from build123d import *

# Parameters (mm, degrees)
F0_R      = 66.728095
F1_DEPTH  = 12.7
F3_DEPTH  = 25.4
F5_DEPTH  = 25.4
F7_DEPTH  = 12.7
F9_DEPTH  = 25.4
F11_DEPTH = 6.35


with BuildPart() as f1:
    # F0 (on Top) → F1 (new body)
    with BuildSketch(Plane.XY):
        with Locations((-8.514826, -3.963798)):
            Circle(F0_R)
    extrude(amount=F1_DEPTH)

    # F2 (on face) → F3 (cut)
    with BuildSketch(Plane.XY.offset(12.7)):
        Polygon((-24.658037, 21.874294), (-35.525352, 38.316716), (-46.980087, 21.874294), align=None)
    extrude(amount=-F3_DEPTH, mode=Mode.SUBTRACT)

    # F4 (on face) → F5 (cut)
    with BuildSketch(Plane.XY.offset(12.7)):
        Polygon((27.306164, 23.048753), (17.029652, 40.372021), (7.633982, 23.048753), align=None)
    extrude(amount=-F5_DEPTH, mode=Mode.SUBTRACT)

    # F6 (on face) → F7 (cut)
    with BuildSketch(Plane.XY.offset(12.7)):
        with BuildLine():
            Line((-25.250863, -24.516826), (-47.612483, -25.613372))
            ThreePointArc((-47.612483, -25.613372), (-7.129461, -49.828593), (32.297611, -23.929598))
            Line((32.297611, -23.929598), (5.287732, -24.516826))
            Line((5.287732, -24.516826), (5.287732, -36.022174))
            Line((5.287732, -36.022174), (-5.854146, -36.568538))
            Line((-5.854146, -36.568538), (-6.470212, -24.005227))
            Line((-6.470212, -24.005227), (-16.903157, -24.516826))
            Line((-16.903157, -24.516826), (-16.49087, -32.924499))
            Line((-16.49087, -32.924499), (-24.818552, -33.332863))
            Line((-24.818552, -33.332863), (-25.250863, -24.516826))
        make_face()
    extrude(amount=-F7_DEPTH, mode=Mode.SUBTRACT)

    # F8 (on face) → F9 (cut)
    with BuildSketch(Plane.XY.offset(12.7)):
        Polygon((-4.40422, -6.606331), (-12.038202, 6.312716), (-19.965798, -6.606331), align=None)
    extrude(amount=-F9_DEPTH, mode=Mode.SUBTRACT)

    # F10 (on Top) → F11 (join)
    with BuildSketch(Plane.XY):
        Polygon((-23.02446, 68.209961), (-25.039101, 60.43921), (0, 60.43921), (-3.453669, 68.209961), align=None)
    extrude(amount=F11_DEPTH)


solid = f1.part
Input: part model. Units: mm. Frame: model coordinates. A direction names the side the tool comes from. Give positions to 0.01 mm unless a question says otherwise; leave off trailing zeros. Order: outer loops, then holes, each group sorted by start corner. A loop starts at its lowest first (then second) coordinate and runs counter-clockwise, first axis right, second up. Notation, with made-up numbers: (-19, -24.5) - (21, -24.5) arc R26 cw to (21, -2.5) - close; hole circle Ø1 at (-15.75, 15). An arc over 180 degrees is marked (long way). Write each question's results on one line, items separated by ' | '.
Item 1: Section A-A (z = 3.75). Return loops of the section in (x, y), and give its area (3 significant figures).
A:
outline: (-24.97, 60.7) arc R66.73 ccw (long way) to (-0.84, 62.32) - (-3.45, 68.21) - (-23.02, 68.21) - close; hole (-47.61, -25.61) arc R44.39 ccw to (32.3, -23.93) - (5.29, -24.52) - (5.29, -36.02) - (-5.85, -36.57) - (-6.47, -24.01) - (-16.9, -24.52) - (-16.49, -32.92) - (-24.82, -33.33) - (-25.25, -24.52) - close; hole (-46.98, 21.87) - (-24.66, 21.87) - (-35.53, 38.32) - close; hole (-19.97, -6.61) - (-4.4, -6.61) - (-12.04, 6.31) - close; hole (7.63, 23.05) - (27.31, 23.05) - (17.03, 40.37) - close | area: 12,400 mm^2
Item 2: Access query for faces 5 (the flat face through (-9, -16, 0)), 6 (the flat face through (-41.173, 30.211, 6.439)). Directions: +Z, -Z, +X, -X, +Y, -Y. A direction counts if a zero-diameter tool reaches every point of the face in a straight line with its end or side. Return the directions, or none.
A:
face 5: -Z, +X, -X, +Y, -Y | face 6: +Z, -Z
Item 3: Section B-B (x = -39). Return loops of the section in (y, z), and give its area (3 significant figures).
A:
outline: (-63.32, 0) - (-37.29, 0) - (-37.29, 12.7) - (-63.32, 12.7) - close; (-25.19, 0) - (21.87, 0) - (21.87, 12.7) - (-25.19, 12.7) - close; (33.33, 0) - (55.39, 0) - (55.39, 12.7) - (33.33, 12.7) - close | area: 1,210 mm^2
Item 4: Material intervals for line 1 along Y through (x, z) = (18, 7.5); line 2 along Y through (x, z) = (-10.5, 3); line 3 along X through (y, z) = (36.5, 6), sorted ascending.
A:
line 1: y = -65.2 to -41.38, -24.24 to 23.05, 38.74 to 57.27 | line 2: y = -70.66 to -49.77, -24.2 to -6.61, 3.71 to 68.21 | line 3: x = -61.57 to -36.79, -34.32 to 14.93, 19.33 to 44.54
Item 5: Contact query for flat-ended pins moving along their axis: pin 1 Ø5 at (x, z) = (-28, 4) entering from -Y; pin 2 Ø6.5 at (x, z) = (-35, 5) entering from +Y; pin 3 Ø2.5 at (x, y) = (-13, 66) entering from +Z. Output: stop coordinate, or through.
A:
pin 1: stops at y = -68.49 | pin 2: stops at y = 58.59 | pin 3: stops at z = 6.35
Item 6: Section C-C (y = -21.5). Return loops of the section in (x, z), and give its area (3 significant figures).
A:
outline: (-72.9, 0) - (55.87, 0) - (55.87, 12.7) - (-72.9, 12.7) - close | area: 1,640 mm^2
Item 7: Section D-D (x = 35). Return loops of the section in (y, z), and give its area (3 significant figures).
A:
outline: (-54.55, 0) - (46.62, 0) - (46.62, 12.7) - (-54.55, 12.7) - close | area: 1,280 mm^2
Item 8: Draft query along X for faces 1 (the flat face through (-25.03, -28.99, 6.44)), 2 (the flat face through (-23.984, 64.509, 3.131)), 3 (the flat face through (-2.127, 65.224, 3.131)), 4 (the flat face through (-0.21, -36.29, 6.44)). Return one class per face: released by +X, released by -X, zero draft, split by the parting line, or undercut.
A:
face 1: undercut | face 2: released by -X | face 3: released by +X | face 4: undercut
